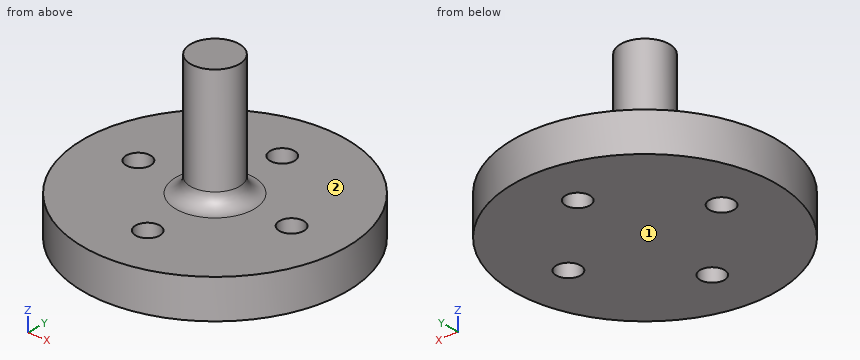
from build123d import *

# Parameters (mm, degrees)
SKETCH1_R           = 27
BOSS_EXTRUDE1_DEPTH = 8
SKETCH2_R           = 2.5
CUT_EXTRUDE1_DEPTH  = 8
SKETCH3_R           = 5
BOSS_EXTRUDE2_DEPTH = 25
FILLET1_R           = 3


with BuildPart() as part:
    # Sketch1 → Boss-Extrude1 (new body)
    with BuildSketch(Plane.XY):
        Circle(SKETCH1_R)
    extrude(amount=BOSS_EXTRUDE1_DEPTH)

    # Sketch2 → Cut-Extrude1 (cut)
    with BuildSketch(Plane.XY.offset(8)):
        with Locations((-16, 0)):
            Circle(SKETCH2_R)
        with Locations((0, 16)):
            Circle(SKETCH2_R)
        with Locations((16, 0)):
            Circle(SKETCH2_R)
        with Locations((0, -16)):
            Circle(SKETCH2_R)
    extrude(amount=-CUT_EXTRUDE1_DEPTH, mode=Mode.SUBTRACT)

    # Sketch3 → Boss-Extrude2 (add)
    with BuildSketch(Plane.XY.offset(8)):
        Circle(SKETCH3_R)
    extrude(amount=BOSS_EXTRUDE2_DEPTH)

    # Fillet1
    fillet1_edges = [part.edges().sort_by_distance(p)[0] for p in [
        (-5, 0, 8),
    ]]
    fillet(fillet1_edges, radius=FILLET1_R)


solid = part.part
CAD build for the part. Positions are in the model's coordinates, mm. Face numbers are marked on the shaded views. A direction names the side the tool comes from. Give positions to 0.01 mm unless a question says otherwise; leave off trailing zeros. Write each loop counter-clockwise with the first axis right and the second up, starting at its lowest first coordinate (ties: lowest second). Pieces come first, ordered by that corner, then holes. Notation, with made-up numbers: (58, 8) - (112, 8) arc R29 cw to (112, 36) - close; hole circle Ø7 at (-39.5, 40.25). An arc over 180 degrees is marked (long way). Put each result on its own line as item: value.
(1) Drop flat-ended pins along their axis: pin 1 Ø1.5 at (x, z) = (9, 4) entering from -Y; pin 2 Ø12 at (x, z) = (-4.5, 15.5) entering from -Y; pin 3 Ø6 at (x, y) = (0, 16) entering from +Z. Give the stop position or say it passes through.
Working result:
pin 1: y = -25.71
pin 2: y = -5
pin 3: z = 8
(2) Wall check: L1, parallel to Y at x = 0, z = 3.5; L2, parallel to Z at x = 6.5, y = -10; L3, parallel to Y at x = 0, z = 15.5. Give the ranges that are in metal, low to high.
Working result:
L1: -27 to -18.5, -13.5 to 13.5, 18.5 to 27
L2: 0 to 8
L3: -5 to 5
(3) Saw through at D-D (z = 14). List the corners of the cut face in (x, y), then the cut area to 3 significant figures.
Working result:
outline: circle Ø10 at (0, 0)
area: 78.5 mm^2
(4) Saw through at B-B (y = -16). List the corners of the cut face in (x, z), then the cut area to 3 significant figures.
Working result:
outline: (-21.75, 0) - (-2.5, 0) - (-2.5, 8) - (-21.75, 8) - close; (2.5, 0) - (21.75, 0) - (21.75, 8) - (2.5, 8) - close
area: 308 mm^2
(5) Saw through at A-A (x = 0). List the corners of the cut face in (y, z).
Working result:
outline: (-27, 0) - (-18.5, 0) - (-18.5, 8) - (-27, 8) - close; (-13.5, 0) - (13.5, 0) - (13.5, 8) - (8, 8) arc R3 cw to (5, 11) - (5, 33) - (-5, 33) - (-5, 11) arc R3 cw to (-8, 8) - (-13.5, 8) - close; (18.5, 0) - (27, 0) - (27, 8) - (18.5, 8) - close
(6) Tool access for the marked faces 1 and 2: list every direction of +Z, -Z, +X, -X, +Y, -Y with a clear straight run to the whole face (end or side of a thin tool).
Working result:
face 1: -Z, +X, -X, +Y, -Y
face 2: +Z
